from build123d import *

# Parameters (mm, degrees)
SKETCH1_W           = 32
SKETCH1_H           = 10
BOSS_EXTRUDE1_DEPTH = 4
SKETCH2_R           = 2.6
CUT_EXTRUDE1_DEPTH  = 10
CUT_EXTRUDE4_DEPTH  = 2
BOSS_EXTRUDE4_DEPTH = 10
SKETCH9_W           = 10
SKETCH9_H           = 14
BOSS_EXTRUDE5_DEPTH = 4
SKETCH10_W          = 10
SKETCH10_H          = 14
BOSS_EXTRUDE6_DEPTH = 4
SKETCH6_R           = 1.75
CUT_EXTRUDE5_DEPTH  = 40
CUT_EXTRUDE6_DEPTH  = 5


with BuildPart() as part:
    # Sketch1 → Boss-Extrude1 (new body)
    with BuildSketch(Plane(origin=(0, 0, 0), x_dir=(1, 0, 0), z_dir=(0, 1, 0))):
        with Locations((-1, -2.382550336)):
            Rectangle(SKETCH1_W, SKETCH1_H)
    extrude(amount=BOSS_EXTRUDE1_DEPTH)

    # Sketch2 → Cut-Extrude1 (cut)
    with BuildSketch(Plane(origin=(0, 4, 0), x_dir=(1, 0, 0), z_dir=(0, 1, 0))):
        with Locations((-9, -2.382550336)):
            Circle(SKETCH2_R)
        with Locations((-1, -2.382550336)):
            Circle(SKETCH2_R)
        with Locations((7, -2.382550336)):
            Circle(SKETCH2_R)
    extrude(amount=-CUT_EXTRUDE1_DEPTH, mode=Mode.SUBTRACT)

    # Sketch3 → Cut-Extrude4 (cut)
    with BuildSketch(Plane.XZ):
        with BuildLine():
            Line((-11.6, 4.070744637), (-11.6, 0.694356034))
            ThreePointArc((-11.6, 0.694356034), (-5.9, 2.382550336), (-11.6, 4.070744637))
        make_face()
        with BuildLine():
            Line((-3.6, 4.070744637), (-3.6, 0.694356034))
            ThreePointArc((-3.6, 0.694356034), (2.1, 2.382550336), (-3.6, 4.070744637))
        make_face()
        with BuildLine():
            Line((4.4, 4.070744637), (4.4, 0.694356034))
            ThreePointArc((4.4, 0.694356034), (10.1, 2.382550336), (4.4, 4.070744637))
        make_face()
    extrude(amount=-CUT_EXTRUDE4_DEPTH, mode=Mode.SUBTRACT)

    # Sketch5 → Boss-Extrude4 (add)
    with BuildSketch(Plane.XZ):
        Polygon((-17, -1.617449664), (-17, -2.617449664), (15, -2.617449664), (15, -1.617449664), (15, 7.382550336), (11, 7.382550336), (11, -1.617449664), (3.5, -1.617449664), (3.5, 7.382550336), (2.5, 7.382550336), (2.5, -1.617449664), (-4.5, -1.617449664), (-4.5, 7.382550336), (-5.5, 7.382550336), (-5.5, -1.617449664), (-12.5, -1.617449664), (-12.5, 7.382550336), (-13, 7.382550336), (-13.5, 7.382550336), (-17, 7.382550336), align=None)
    extrude(amount=BOSS_EXTRUDE4_DEPTH)

    # Sketch9 → Boss-Extrude5 (add)
    with BuildSketch(Plane(origin=(15, 0, 0), x_dir=(0, 0, -1), z_dir=(1, 0, 0))):
        with Locations((-2.382550336, -3)):
            Rectangle(SKETCH9_W, SKETCH9_H)
    extrude(amount=BOSS_EXTRUDE5_DEPTH)

    # Sketch10 → Boss-Extrude6 (add)
    with BuildSketch(Plane.ZY.offset(17)):
        with Locations((2.382550336, -3)):
            Rectangle(SKETCH10_W, SKETCH10_H)
    extrude(amount=BOSS_EXTRUDE6_DEPTH)

    # Sketch6 → Cut-Extrude5 (cut)
    with BuildSketch(Plane.XZ.offset(10)):
        with Locations((-16.75, 2.382550336)):
            Circle(SKETCH6_R)
        with Locations((15, 2.382550336)):
            Circle(SKETCH6_R)
    extrude(amount=-CUT_EXTRUDE5_DEPTH, mode=Mode.SUBTRACT)

    # Sketch8 → Cut-Extrude6 (cut)
    with BuildSketch(Plane.XZ.offset(10)):
        Polygon((-16.839532769, 5.556714354), (-19.543673061, 3.892094692), (-19.454140291, 0.717930674), (-16.660467231, -0.791613683), (-13.956326939, 0.873005979), (-14.045859709, 4.047169998), align=None)
        Polygon((15, 5.557976816), (12.25, 3.970263576), (12.25, 0.794837095), (15, -0.792876145), (17.75, 0.794837095), (17.75, 3.970263576), align=None)
    extrude(amount=-CUT_EXTRUDE6_DEPTH, mode=Mode.SUBTRACT)


solid = part.part
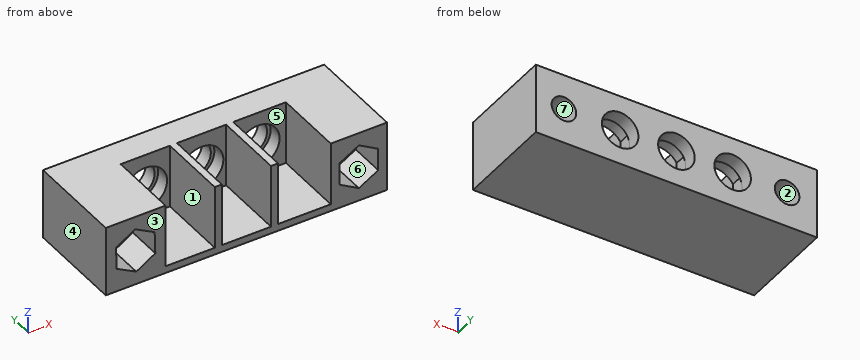
Could you check a few things on this model? Use its own coordinates, in mm. Face numbers are marked on the shaded views. A direction names the side the tool comes from. Round coordinates to 2 decimals unless told otherwise and drop trailing zeros. Write each loop counter-clockwise with the first axis right and the second up, starting at its lowest first coordinate (ties: lowest second). Pieces come first, ordered by that corner, then holes. Notation, with made-up numbers: (-22, 57) - (29, 57) arc R21 cw to (29, 64) - close; hole circle Ø6 at (9, 70). An arc over 180 degrees is marked (long way). Put each result on its own line as item: value. Start each with the question number.
(1) I want a section at C-C, the plane y = -5.5. Please give me the cut outline in (x, z), plus the area to 3 significant figures.
(2) I want a section at D-D, the plane y = 1. Please give me the cut outline in (x, z), plus the area to 3 significant figures.
(3) Thinking about a two-plate mould opening in X: for the marked faces 1, 2, 3 and 4, which applies, released by +X, released by -X, zero draft, split by the parting line, or undercut?
(4) Will this pin go through, and if not, where does the flat tip stop? pin 1 (5.5 mm diameter, centred on x = -9, z = 2.38, fed in from -Y).
(5) I want a section at A-A, the plane x = 7. Please give me the cut outline in (y, z), plus the area to 3 significant figures.
(6) I want a section at B-B, the plane z = -1.25. Please give me the cut outline in (x, y), plus the area to 3 significant figures.
(7) I need wall thicknesses on probe 1 along X at (y, z) = (-0.5, -0.25); probe 2 along Z at (x, y) = (-9, 0.65); probe 3 along Z at (x, y) = (-16.75, 0). Which ranges of each line are inside material? Lowest first, please.
(8) For the marked faces 5, 6 and 7, which set-ups out of +Z, -Z, +X, -X, +Y, -Y let a thin tool reach every point of the face, with its end or its side?
Here are the results:
1. outline: (-21, -2.62) - (19, -2.62) - (19, 7.38) - (11, 7.38) - (11, -1.62) - (3.5, -1.62) - (3.5, 7.38) - (2.5, 7.38) - (2.5, -1.62) - (-4.5, -1.62) - (-4.5, 7.38) - (-5.5, 7.38) - (-5.5, -1.62) - (-12.5, -1.62) - (-12.5, 7.38) - (-21, 7.38) - close; hole (-19.54, 3.89) - (-19.45, 0.72) - (-16.66, -0.79) - (-13.96, 0.87) - (-14.05, 4.05) - (-16.84, 5.56) - close; hole (12.25, 0.79) - (15, -0.79) - (17.75, 0.79) - (17.75, 3.97) - (15, 5.56) - (12.25, 3.97) - close
1. area: 154 mm^2
2. outline: (-21, -2.62) - (19, -2.62) - (19, 7.38) - (-21, 7.38) - close; hole circle Ø3.5 at (-16.75, 2.38); hole (-11.6, 0.69) arc R3.1 ccw (long way) to (-11.6, 4.07) - close; hole (-3.6, 0.69) arc R3.1 ccw (long way) to (-3.6, 4.07) - close; hole (4.4, 0.69) arc R3.1 ccw (long way) to (4.4, 4.07) - close; hole circle Ø3.5 at (15, 2.38)
2. area: 294 mm^2
3. face 1: undercut
3. face 2: undercut
3. face 3: zero draft
3. face 4: released by -X
4. pin 1: stops at y = 0
5. outline: (-10, -2.62) - (4, -2.62) - (4, -0.22) - (2, -0.22) - (2, -0.72) - (0, -0.72) - (0, -1.62) - (-10, -1.62) - close; (0, 5.48) - (2, 5.48) - (2, 4.98) - (4, 4.98) - (4, 7.38) - (0, 7.38) - close
5. area: 27.2 mm^2
6. outline: (-21, -10) - (-12.5, -10) - (-12.5, 0) - (-5.5, 0) - (-5.5, -10) - (-4.5, -10) - (-4.5, 0) - (2.5, 0) - (2.5, -10) - (3.5, -10) - (3.5, 0) - (11, 0) - (11, -10) - (19, -10) - (19, 4) - (-21, 4) - close
6. area: 345 mm^2
7. probe 1: x = -21 to -12.5, -5.5 to -4.5, 2.5 to 3.5, 11 to 19
7. probe 2: z = -2.62 to -0.72, 5.48 to 7.38
7. probe 3: z = -2.62 to 0.63, 4.13 to 7.38
8. face 5: +Z, -Y
8. face 6: -Y
8. face 7: +Y, -Y
